The model under review builds one solid part; all positions refer to its coordinate system, in mm. Give positions to 0.01 mm unless a question says otherwise; leave off trailing zeros. Order: outer loops, then holes, each group sorted by start corner. A loop starts at its lowest first (then second) coordinate and runs counter-clockwise, first axis right, second up. Notation, with made-up numbers: M 65,-6 L 106,-6 A26 cw 106,26 Z; hole C 19,49.25 d1. An arc over 180 degrees is marked long. One line per question, with ' | ' between items. Start each with the question number.
1. The part is to be moulded in two halves that separate along X. For faces 1 (the face through (0, 16, 2)), 2 (the face through (74, 32, 2)), 3 (the face through (15.472, 13.893, 2.453)), say which applies: +X half, -X half, draft (parallel to the pull), parting line (faces both ways), or undercut.
2. Insertion check: P1, Ø8, axis at x = 68.5, y = 16.5, coming from the +Z side. The pin has a flat end and moves straight along its axis. Give the tip position at first contact, or say it passes through.
3. Wall thickness on L1, parallel to X at y = 16, z = 3.85; L2, parallel to X at y = 12.5, z = 3.8; L3, parallel to Y at x = 68, z = 4.05: over which ranges is each line inside the solid? List them lowest first.
4. We need section A-A on z = 3.6. Write out the cut boundary in (x, y).
```python
from build123d import *

# Parameters (mm, degrees)
ESQUISSE1_W                 = 151
ESQUISSE1_H                 = 32
BOSS_EXTRU_1_DEPTH          = 5
D_GAGEMENT_M101_D           = 11
D_GAGEMENT_M101_DEPTH       = 37
D_GAGEMENT_M101_CSINK_D     = 11.05
D_GAGEMENT_M101_CSINK_ANGLE = 90
D_GAGEMENT_M101_TIP         = 3.304733405


with BuildPart() as part:
    # Esquisse1 → Boss.-Extru.1 (new body)
    with BuildSketch(Plane.XY):
        with Locations((75.5, 16)):
            Rectangle(ESQUISSE1_W, ESQUISSE1_H)
    extrude(amount=BOSS_EXTRU_1_DEPTH)

    # Dégagement M101
    with Locations(Plane(origin=(20.552465295, 16, 5), x_dir=(1, 0, 0), z_dir=(0, 0, 1))):
        with Locations((0, 0), (48.398815016, 0), (110.018769744, 0)):
            CounterSinkHole(D_GAGEMENT_M101_D / 2, D_GAGEMENT_M101_CSINK_D / 2, depth=D_GAGEMENT_M101_DEPTH, counter_sink_angle=D_GAGEMENT_M101_CSINK_ANGLE)
            with Locations((0, 0, -(D_GAGEMENT_M101_DEPTH + D_GAGEMENT_M101_TIP / 2))):  # 118° drill point
                Cone(0, D_GAGEMENT_M101_D / 2, D_GAGEMENT_M101_TIP, mode=Mode.SUBTRACT)


solid = part.part
```
Entries:
1) face 1: -X half | face 2: draft | face 3: undercut
2) P1: passes through
3) L1: x = 0 to 15.05, 26.05 to 63.45, 74.45 to 125.07, 136.07 to 151 | L2: x = 0 to 16.31, 24.8 to 64.71, 73.19 to 126.33, 134.81 to 151 | L3: y = 0 to 10.58, 21.42 to 32
4) outline: M 0,0 L 151,0 L 151,32 L 0,32 Z; hole C 20.55,16 d11; hole C 68.95,16 d11; hole C 130.57,16 d11
